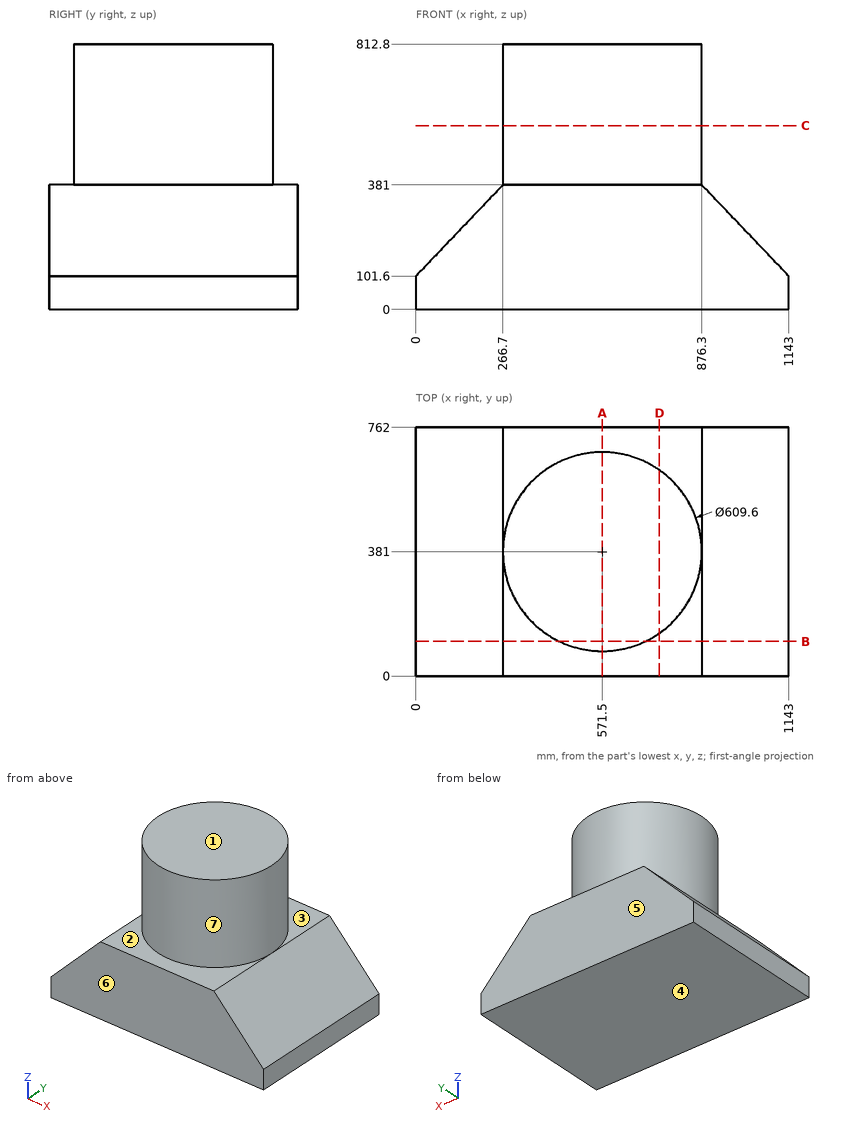
The drawing under review shows one solid part. Ordinate dimensions are in mm from its lowest x, y, z. A direction names the side the tool comes from. Coordinates: 2 decimals unless noted, no trailing zeros. Write each loop counter-clockwise with the first axis right and the second up, starting at its lowest first coordinate (ties: lowest second). Pieces come first, ordered by that corner, then holes. Notation, with made-up numbers: (-32.5, 56.25) -> (-9.5, 56.25) arc R6 ccw to (-9.5, 63.25) -> close; hole circle Ø1 at (51.25, 43.5). An arc over 180 degrees is marked (long way). One line per item, written item: value. Start each with the question number.
Q1. Add section D-D, the plane x = 746.5. Give the boundary of the cut face in (y, z), then the cut area to 3 significant figures.
Q2. For the marked faces 1, 2 and 3, list the 3-axis set-ups (+Z, -Z, +X, -X, +Y, -Y) from which the entire face can be reached by the end or side of a thin tool; tool diameter is ignored.
Q3. Add section B-B, the plane y = 106. Give the boundary of the cut face in (x, z).
Q4. The part is to be moulded in two halves that separate along Y. For the marked faces 4, 5, 6 and 7, say which applies: +Y half, -Y half, draft (parallel to the pull), parting line (faces both ways), or undercut.
Q5. Add section C-C, the plane z = 563. Give the boundary of the cut face in (x, y).
Q6. To check wall thickness, follow probe 1 along Z at (x, y) = (821.5, 613.5); probe 2 along X at (y, z) = (314, 181); probe 3 along X at (y, z) = (128, 586). State the ranges of each line that lie inside material, in increasing order.
Q7. Clearance check with flat-ended pins moving along their axes: P1, Ø10, axis at y = 595, z = 310, coming from the +X side; P2, Ø1, axis at x = 323.5, z = 402.5, coming from the -Y side; P3, Ø5, axis at y = 654.5, z = 621.5, coming from the +X side. State where each tip first meets the part, or that it passes through.
Q8. Add section A-A, the plane x = 571.5. Give the boundary of the cut face in (y, z).
Response:
1. outline: (0, 0) -> (762, 0) -> (762, 381) -> (630.56, 381) -> (630.56, 812.8) -> (131.44, 812.8) -> (131.44, 381) -> (0, 381) -> close
1. area: 506,000 mm²
2. face 1: +Z, +X, -X, +Y, -Y
2. face 2: +Z, -Y
2. face 3: +Z, +Y
3. outline: (0, 0) -> (1143, 0) -> (1143, 101.6) -> (876.3, 381) -> (702.95, 381) -> (702.95, 812.8) -> (440.05, 812.8) -> (440.05, 381) -> (266.7, 381) -> (0, 101.6) -> close
4. face 4: draft
4. face 5: +Y half
4. face 6: -Y half
4. face 7: parting line
5. outline: circle Ø609.6 at (571.5, 381)
6. probe 1: 0 to 381
6. probe 2: 75.79 to 1067.21
6. probe 3: 401.52 to 741.48
7. P1: x = 948.85
7. P2: y = 203.1
7. P3: x = 711.01
8. outline: (0, 0) -> (762, 0) -> (762, 381) -> (685.8, 381) -> (685.8, 812.8) -> (76.2, 812.8) -> (76.2, 381) -> (0, 381) -> close
